The listing builds one solid part. Answer for the finished solid, in the listing's coordinates (mm). Face numbers are marked on the shaded views. A direction names the side the tool comes from. Coordinates: 2 decimals unless noted, no trailing zeros. Loops run counter-clockwise (first coordinate to the right, second up) from the corner with the lowest first, then second, coordinate; pieces in that order, holes last. Notation, with made-up numbers: (79.25, -31.75) - (136.25, -31.75) arc R20 ccw to (136.25, 3.25) - close; hole circle Ø9 at (30.5, 9). An arc over 180 degrees is marked (long way). Put each result on its own line as item: value.
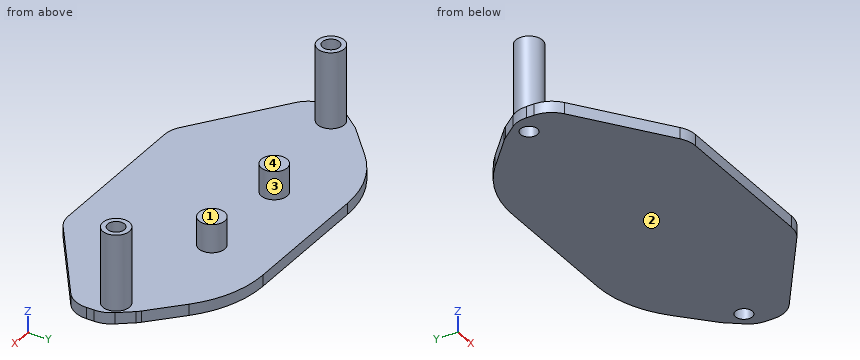
```python
from build123d import *

# Parameters (mm, degrees)
ESQUISSE1_R             = 1.5
BOSS_EXTRU_3_DEPTH      = 2
BOSS_EXTRU_4_START      = -53.32
ESQUISSE2_R             = 2.3
BOSS_EXTRU_4_DEPTH      = 5
ESQUISSE3_R             = 1.5
ENL_V_MAT_EXTRU_1_DEPTH = 10
ESQUISSE4_R             = 2.37
ESQUISSE4_R_2           = 1.5
BOSS_EXTRU_5_DEPTH      = 13.5


with BuildPart() as part:
    # Esquisse1 → Boss.-Extru.3 (new body)
    with BuildSketch(Plane.XY):
        with BuildLine():
            Line((31.640550531, -4.887241018), (16.450544828, -15.819470843))
            ThreePointArc((16.450544828, -15.819470843), (15.064222472, -16.51996197), (13.529826111, -16.761219719))
            Line((13.529826111, -16.761219719), (-13.529826111, -16.761219719))
            ThreePointArc((-13.529826111, -16.761219719), (-15.064222472, -16.51996197), (-16.450544828, -15.819470843))
            Line((-16.450544828, -15.819470843), (-31.640550531, -4.887241018))
            ThreePointArc((-31.640550531, -4.887241018), (-33.169752802, -3.108946738), (-33.719831815, -0.828989895))
            Line((-33.719831815, -0.828989895), (-33.719831815, 0.549989061))
            ThreePointArc((-33.719831815, 0.549989061), (-33.448369589, 2.175083064), (-32.663459607, 3.623716413))
            Line((-32.663459607, 3.623716413), (-30.727499402, 6.107575779))
            ThreePointArc((-30.727499402, 6.107575779), (-30.464326323, 6.418261685), (-30.17674656, 6.706504084))
            Line((-30.17674656, 6.706504084), (-24.719522272, 11.748000297))
            ThreePointArc((-24.719522272, 11.748000297), (-18.785145606, 15.463312907), (-11.905042981, 16.761219719))
            Line((-11.905042981, 16.761219719), (11.905042981, 16.761219719))
            ThreePointArc((11.905042981, 16.761219719), (18.785145606, 15.463312907), (24.719522272, 11.748000297))
            Line((24.719522272, 11.748000297), (30.17674656, 6.706504084))
            ThreePointArc((30.17674656, 6.706504084), (30.464326323, 6.418261685), (30.727499402, 6.107575779))
            Line((30.727499402, 6.107575779), (32.663459607, 3.623716413))
            ThreePointArc((32.663459607, 3.623716413), (33.448369589, 2.175083064), (33.719831815, 0.549989061))
            Line((33.719831815, 0.549989061), (33.719831815, -0.828989895))
            ThreePointArc((33.719831815, -0.828989895), (33.169752802, -3.108946738), (31.640550531, -4.887241018))
        make_face()
        with Locations((-30.225692015, 2.268354752)):
            Circle(ESQUISSE1_R, mode=Mode.SUBTRACT)
        with Locations((30.225692015, 2.268354752)):
            Circle(ESQUISSE1_R, mode=Mode.SUBTRACT)
    extrude(amount=BOSS_EXTRU_3_DEPTH)

    # Esquisse2 → Boss.-Extru.4 (add)
    with BuildSketch(Plane.XY.offset(55.32).offset(BOSS_EXTRU_4_START)):
        with Locations((-8.781978503, 5.736063319)):
            Circle(ESQUISSE2_R)
        with Locations((8.782063878, 5.73606332)):
            Circle(ESQUISSE2_R)
    extrude(amount=BOSS_EXTRU_4_DEPTH)

    # Esquisse3 → Enlèv. mat.-Extru.1 (cut)
    with BuildSketch(Plane(origin=(0, 0, 0), x_dir=(-1, 0, 0), z_dir=(0, 0, -1))):
        with Locations((60.239561974, 19.762236701)):
            Circle(ESQUISSE3_R)
        with Locations((-29.955535999, 19.762236701)):
            Circle(ESQUISSE3_R)
    extrude(amount=-ENL_V_MAT_EXTRU_1_DEPTH, mode=Mode.SUBTRACT)

    # Esquisse4 → Boss.-Extru.5 (add)
    # profile 1 of 2: a face of its own
    with BuildSketch(Plane.XY.offset(2)):
        with Locations((30.225692015, 2.268354752)):
            Circle(ESQUISSE4_R)
        with Locations((30.225692015, 2.268354752)):
            Circle(ESQUISSE4_R_2, mode=Mode.SUBTRACT)
    # profile 2 of 2: a face of its own
    with BuildSketch(Plane.XY.offset(2)):
        with Locations((-30.225692015, 2.268354752)):
            Circle(ESQUISSE4_R)
        with Locations((-30.225692015, 2.268354752)):
            Circle(ESQUISSE4_R_2, mode=Mode.SUBTRACT)
    extrude(amount=BOSS_EXTRU_5_DEPTH)


solid = part.part
```
1) Each of these flat-tipped pins is pushed along its axis until it touches: pin 1 (8 mm diameter, centred on x = -3, y = -11.5, fed in from +Z); pin 2 (5 mm diameter, centred on x = -30.23, y = 2.27, fed in from +Z); pin 3 (2 mm diameter, centred on y = 2.5, z = 4, fed in from -X); pin 4 (3.5 mm diameter, centred on x = -8.5, y = 6, fed in from +Z). Where does it stop, or does it pass through?
Found:
pin 1: stops at z = 2
pin 2: stops at z = 15.5
pin 3: stops at x = -32.6
pin 4: stops at z = 7
2) Straight lines are drawn through the part: L1, parallel to X at y = 1.5, z = 8.25; L2, parallel to X at y = 3.5, z = 7.5; L3, parallel to Z at x = 0, y = -2.5. For each, find the intervals that lie inside material, in ascending order. Write a range as [from, to].
Found:
L1: x = [-32.47, -31.51], [-28.94, -27.98], [27.98, 28.94], [31.51, 32.47]
L2: x = [-32.25, -31.08], [-29.37, -28.2], [28.2, 29.37], [31.08, 32.25]
L3: z = [0, 2]
3) For a pull along X with two mould halves and no side action, classify the marked faces 1 and 2 as pulls with the +X half, pulls with the -X half, needs draft (parallel to the pull), parting line crosses it, or undercut.
Found:
face 1: undercut
face 2: needs draft
4) The part is cut by section D-D (y = 13.5). Give the vertices of the cut face in (x, z).
Found:
outline: (-22.51, 0) - (22.51, 0) - (22.51, 2) - (-22.51, 2) - close
5) The part is cut by section B-B (x = 5). Give the vertices of the cut face in (y, z), and give its area (3 significant figures).
Found:
outline: (-16.76, 0) - (16.76, 0) - (16.76, 2) - (-16.76, 2) - close
area: 67.0 mm^2
6) For the marked faces 3 and 4, determine the directions among +Z, -Z, +X, -X, +Y, -Y from which every point of the face is accessible in a straight line to the end or side of a thin tool.
Found:
face 3: +Z
face 4: +Z, +Y, -Y
7) The part is cut by section A-A (z = 4.75). Give the vertices of the cut face in (x, y).
Found:
outline: circle Ø4.74 at (-30.23, 2.27); circle Ø4.6 at (-8.78, 5.74); circle Ø4.6 at (8.78, 5.74); circle Ø4.74 at (30.23, 2.27); hole circle Ø3 at (-30.23, 2.27); hole circle Ø3 at (30.23, 2.27)
8) The part is cut by section C-C (z = 7.75). Give the vertices of the cut face in (x, y).
Found:
outline: circle Ø4.74 at (-30.23, 2.27); circle Ø4.74 at (30.23, 2.27); hole circle Ø3 at (-30.23, 2.27); hole circle Ø3 at (30.23, 2.27)
